Check sheet for the drawn part. Datum: minimum x, y, z corner. Units: mm. A direction names the side the tool comes from. Round coordinates to 2 decimals unless told otherwise and drop trailing zeros. Order: outer loops, then holes, each group sorted by start corner. A loop starts at its lowest first (then second) coordinate and runs counter-clockwise, first axis right, second up. Notation, with made-up numbers: (41.5, 20) - (86.5, 20) arc R23 ccw to (86.5, 28) - close; hole circle Ø4 at (-21, 49.25). An arc over 180 degrees is marked (long way). Write each question's results on one line, items separated by ' | '.
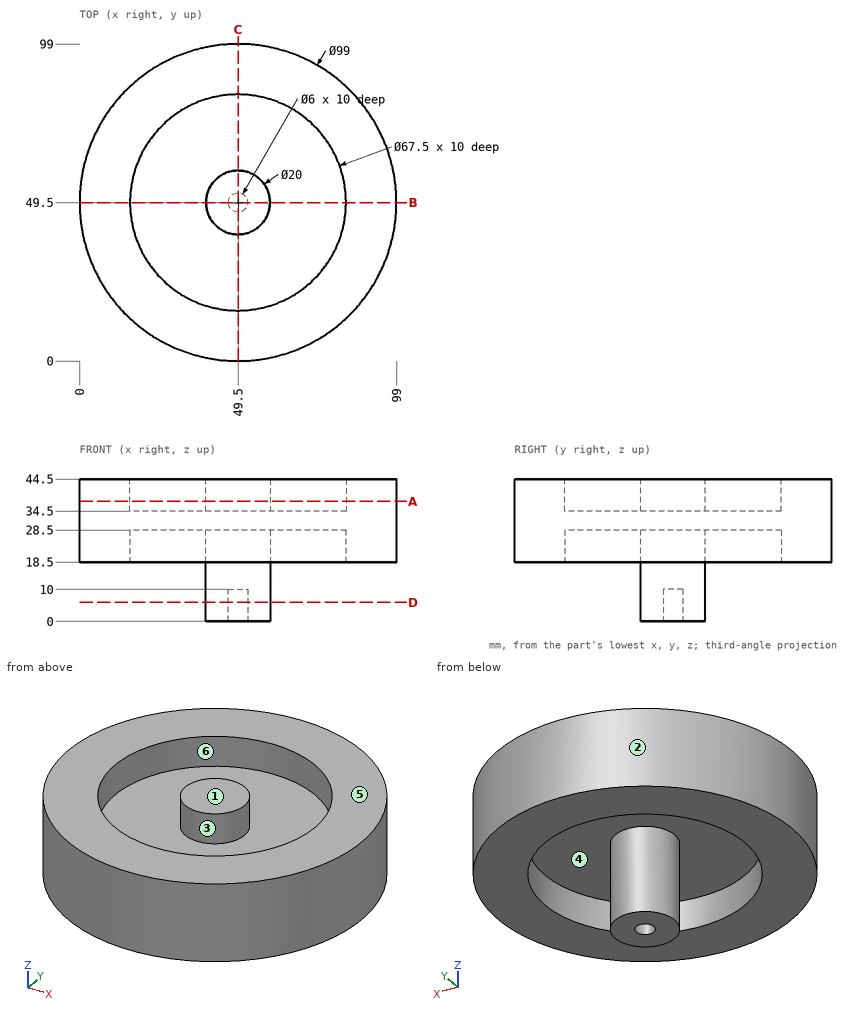
(1) Section check B-B (y = 49.5). Record the cut outline in (x, z), then the cut area to 3 significant figures.
Answers follow:
outline: (0, 18.5) - (15.75, 18.5) - (15.75, 28.5) - (39.5, 28.5) - (39.5, 0) - (46.5, 0) - (46.5, 10) - (52.5, 10) - (52.5, 0) - (59.5, 0) - (59.5, 28.5) - (83.25, 28.5) - (83.25, 18.5) - (99, 18.5) - (99, 44.5) - (83.25, 44.5) - (83.25, 34.5) - (59.5, 34.5) - (59.5, 44.5) - (39.5, 44.5) - (39.5, 34.5) - (15.75, 34.5) - (15.75, 44.5) - (0, 44.5) - close | area: 1,930 mm²
(2) Access from +Z, -Z, +X, -X, +Y, -Y to the whole of each face (thin tool, end or side, straight path). Record for the marked faces 4, 5 and 6.
Answers follow:
face 4: -Z | face 5: +Z, +X, -X, +Y, -Y | face 6: +Z
(3) Section check A-A (z = 37.5). Record the cut outline in (x, y), then the cut area to 3 significant figures.
Answers follow:
outline: circle Ø99 at (49.5, 49.5); circle Ø20 at (49.5, 49.5); hole circle Ø67.5 at (49.5, 49.5) | area: 4,430 mm²
(4) Material ranges on line 1 (Y direction, x = 49, z = 37); line 2 (Y direction, x = 49.5, z = 5.25), recorded low to high.
Answers follow:
line 1: 0 to 15.75, 39.51 to 59.49, 83.25 to 99 | line 2: 39.5 to 46.5, 52.5 to 59.5
(5) Draft check along X on the marked faces 1, 2 and 3. Enter one of: released by +X, released by -X, zero draft, split by the parting line, or undercut.
Answers follow:
face 1: zero draft | face 2: split by the parting line | face 3: undercut
(6) Section check D-D (z = 6). Record the cut outline in (x, y).
Answers follow:
outline: circle Ø20 at (49.5, 49.5); hole circle Ø6 at (49.5, 49.5)
(7) Depth check by flat-ended pin: pin 1 Ø7 at (x, y) = (49.5, 49.5) entering from -Z; pin 2 Ø4 at (x, y) = (61.5, 35) entering from -Z; pin 3 Ø1.8 at (x, y) = (49, 50.5) entering from -Z; pin 4 Ø2 at (y, z) = (37, 26.5) entering from -X. Enter the tip coordinate at first touch or a pass-through.
Answers follow:
pin 1: z = 0 | pin 2: z = 28.5 | pin 3: z = 10 | pin 4: x = 1.35
